Geometry check sheet. Reference: the model listing, model coordinates, mm. Face numbers are marked on the shaded views. A direction names the side the tool comes from. Give positions to 0.01 mm unless a question says otherwise; leave off trailing zeros. Write each loop counter-clockwise with the first axis right and the second up, starting at its lowest first coordinate (ties: lowest second). Pieces come first, ordered by that corner, then holes. Notation, with made-up numbers: (22, 32) -> (67, 32) arc R23 ccw to (67, 49) -> close; hole circle Ø3 at (59.25, 61). An arc over 180 degrees is marked (long way). Use a Markdown table: item, result. Add a question column.
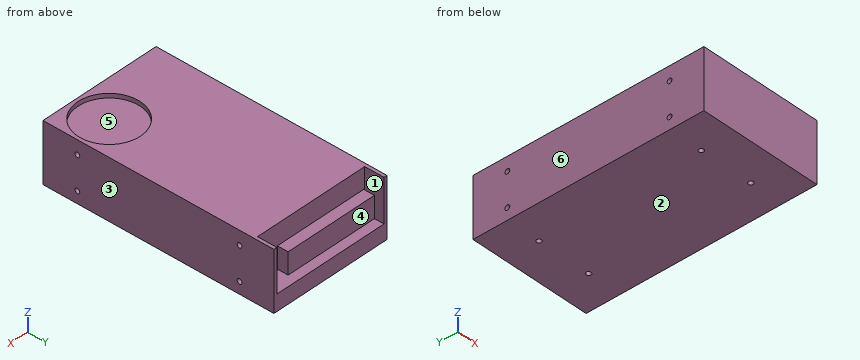
from build123d import *

# Parameters (mm, degrees)
SKETCH1_W           = 114
SKETCH1_H           = 215
BOSS_EXTRUDE1_DEPTH = 55
SKETCH2_W           = 108
SKETCH2_H           = 18
CUT_EXTRUDE1_DEPTH  = 40
SKETCH3_W           = 87
SKETCH3_H           = 20
BOSS_EXTRUDE2_DEPTH = 10
SKETCH4_R           = 29
CUT_EXTRUDE3_DEPTH  = 4
SKETCH5_R           = 2.25
CUT_EXTRUDE4_DEPTH  = 15
SKETCH6_R           = 2.25
CUT_EXTRUDE5_DEPTH  = 167.063993689


with BuildPart() as part:
    # Sketch1 → Boss-Extrude1 (new body)
    with BuildSketch(Plane.XY):
        Rectangle(SKETCH1_W, SKETCH1_H)
    extrude(amount=BOSS_EXTRUDE1_DEPTH)

    # Sketch2 → Cut-Extrude1 (cut)
    with BuildSketch(Plane.XY.offset(55)):
        with Locations((0, 98.5)):
            Rectangle(SKETCH2_W, SKETCH2_H)
    extrude(amount=-CUT_EXTRUDE1_DEPTH, mode=Mode.SUBTRACT)

    # Sketch3 → Boss-Extrude2 (add)
    with BuildSketch(Plane(origin=(0, 89.5, 0), x_dir=(1, 0, 0), z_dir=(0, 1, 0))):
        with Locations((-9.5, -26)):
            Rectangle(SKETCH3_W, SKETCH3_H)
    extrude(amount=BOSS_EXTRUDE2_DEPTH)

    # Sketch4 → Cut-Extrude3 (cut)
    with BuildSketch(Plane.XY.offset(55)):
        with Locations((25, -75.5)):
            Circle(SKETCH4_R)
    extrude(amount=-CUT_EXTRUDE3_DEPTH, mode=Mode.SUBTRACT)

    # Sketch5 → Cut-Extrude4 (cut)
    with BuildSketch(Plane(origin=(0, 0, 0), x_dir=(-1, 0, 0), z_dir=(0, 0, -1))):
        with Locations((-25, 75.5)):
            Circle(SKETCH5_R)
        with Locations((25, 75.5)):
            Circle(SKETCH5_R)
        with Locations((25, -75.5)):
            Circle(SKETCH5_R)
        with Locations((-25, -75.5)):
            Circle(SKETCH5_R)
    extrude(amount=-CUT_EXTRUDE4_DEPTH, mode=Mode.SUBTRACT)

    # Sketch6 → Cut-Extrude5 (cut, through all)
    with BuildSketch(Plane.ZY.offset(57)):
        with Locations(Location((11, 75.5, 0), (0, 0, 270))):
            Circle(SKETCH6_R)
        with Locations(Location((42, 75.5, 0), (0, 0, 270))):
            Circle(SKETCH6_R)
        with Locations(Location((42, -75.5, 0), (0, 0, 270))):
            Circle(SKETCH6_R)
        with Locations(Location((11, -75.5, 0), (0, 0, 270))):
            Circle(SKETCH6_R)
    extrude(amount=-CUT_EXTRUDE5_DEPTH, mode=Mode.SUBTRACT)


solid = part.part
1) Draft check along X on the marked faces 1, 2 and 3. Enter one of: +X half, -X half, draft (parallel to the pull), parting line (faces both ways), or undercut.
2) Sectioned sample at A-A, the plane z = 42. Enter the section's corners in (x, y).
3) Gauge pin test, flat ends, axial feed: P1, Ø1, axis at x = 42.5, y = -69.5, coming from the -Z side; P2, Ø3.5, axis at x = -25, y = -75.5, coming from the -Z side; P3, Ø12, axis at x = -16, z = 38.5, coming from the +Y side. Record the tip position at first contact, or that the pin passes through.
4) Tool access check on the marked faces 4, 5 and 6. Record the directions out of +Z, -Z, +X, -X, +Y, -Y that give a thin tool (end or side, any length) a straight path to the whole face; none if there is none.
5) Sectioned sample at C-C, the plane x = 46. Enter the section's corners in (y, z), and give its area (3 significant figures).
6) Sectioned sample at D-D, the plane z = 28. Enter the section's corners in (x, y), and give its area (3 significant figures).
7) Sectioned sample at B-B, the plane y = 75.5. Enter the section's corners in (x, z), and give its area (3 significant figures).
8) Material ranges on probe 1 along Y at (x, z) = (-25, 7); probe 2 along Z at (x, y) = (-34, 96); probe 3 along Y at (x, z) = (8.5, 42.5), recorded low to high. Write a range as [from, to].
Check values:
| question | item | result |
|---|---|---|
| 1 | face 1 | undercut |
| 1 | face 2 | draft |
| 1 | face 3 | +X half |
| 2 | outline | (-57, -107.5) -> (57, -107.5) -> (57, -77.75) -> (-57, -77.75) -> close; (-57, -73.25) -> (57, -73.25) -> (57, 73.25) -> (-57, 73.25) -> close; (-57, 77.75) -> (57, 77.75) -> (57, 107.5) -> (54, 107.5) -> (54, 89.5) -> (-54, 89.5) -> (-54, 107.5) -> (-57, 107.5) -> close |
| 3 | P1 | z = 0 |
| 3 | P2 | z = 15 |
| 3 | P3 | y = 99.5 |
| 4 | face 4 | +Z, +Y |
| 4 | face 5 | +Z |
| 4 | face 6 | +Z, -Z, -X, +Y, -Y |
| 5 | outline | (-107.5, 0) -> (107.5, 0) -> (107.5, 15) -> (89.5, 15) -> (89.5, 55) -> (-55.5, 55) -> (-55.5, 51) -> (-95.5, 51) -> (-95.5, 55) -> (-107.5, 55) -> close; hole circle Ø4.5 at (-75.5, 11); hole circle Ø4.5 at (-75.5, 42); hole circle Ø4.5 at (75.5, 11); hole circle Ø4.5 at (75.5, 42) |
| 5 | area | 10,900 mm² |
| 6 | outline | (-57, -107.5) -> (57, -107.5) -> (57, 107.5) -> (54, 107.5) -> (54, 89.5) -> (34, 89.5) -> (34, 99.5) -> (-53, 99.5) -> (-53, 89.5) -> (-54, 89.5) -> (-54, 107.5) -> (-57, 107.5) -> close |
| 6 | area | 23,400 mm² |
| 7 | outline | (-57, 0) -> (-27.25, 0) -> (-27.25, 8.75) -> (-57, 8.75) -> close; (-57, 13.25) -> (-27.25, 13.25) -> (-27.25, 15) -> (-22.75, 15) -> (-22.75, 13.25) -> (22.75, 13.25) -> (22.75, 15) -> (27.25, 15) -> (27.25, 13.25) -> (57, 13.25) -> (57, 39.75) -> (-57, 39.75) -> close; (-57, 44.25) -> (57, 44.25) -> (57, 55) -> (-57, 55) -> close; (-22.75, 0) -> (22.75, 0) -> (22.75, 8.75) -> (-22.75, 8.75) -> close; (27.25, 0) -> (57, 0) -> (57, 8.75) -> (27.25, 8.75) -> close |
| 7 | area | 5,150 mm² |
| 8 | probe 1 | [-107.5, -77.75], [-73.25, 73.25], [77.75, 107.5] |
| 8 | probe 2 | [0, 15], [16, 36] |
| 8 | probe 3 | [-107.5, -77.69], [-73.31, 73.31], [77.69, 89.5] |
